Work out the finished part from the listing and answer in its coordinate system (mm). Face numbers are marked on the shaded views. Round coordinates to 2 decimals unless told otherwise and drop trailing zeros. Order: outer loops, then holes, each group sorted by start corner. A loop starts at its lowest first (then second) coordinate and runs counter-clockwise, first axis right, second up. Notation, with made-up numbers: (76, -18) - (96, -18) arc R22 ccw to (96, 15) - close; hole circle Ø8 at (59.5, 9). An arc over 180 degrees is marked (long way). Put each result on its own line as item: value.
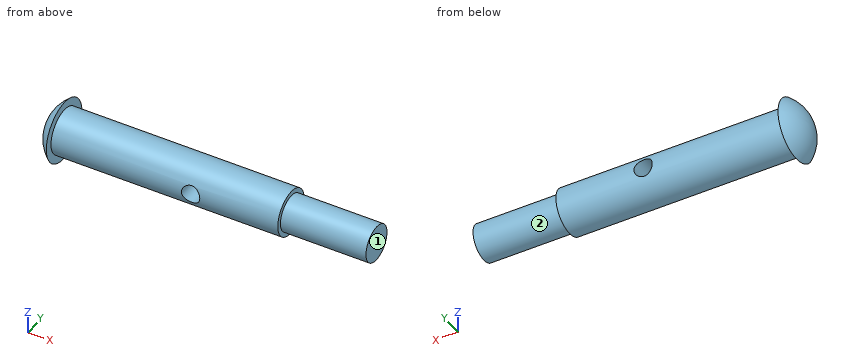
```python
from build123d import *

# Parameters (mm, degrees)
SKETCH4_R               = 0.9906
CUT_EXTRUDE1_DEPTH      = 4.3274
CUT_EXTRUDE1_DEPTH_BACK = 4.3274


with BuildPart() as part:
    # Sketch1 → Revolve1 (revolve)
    with BuildSketch(Plane.XY):
        with BuildLine():
            Line((0, 3.3274), (0, 2.45745))
            Line((0, 2.45745), (24.511, 2.45745))
            Line((24.511, 2.45745), (24.511, 1.96215))
            Line((24.511, 1.96215), (33.7566, 1.96215))
            Line((33.7566, 1.96215), (33.7566, 0))
            Line((33.7566, 0), (-1.651, 0))
            ThreePointArc((-1.651, 0), (-1.21556162, 1.857242025), (0, 3.3274))
        make_face()
    revolve(axis=Axis((0, 0, 0), (1, 0, 0)))

    # Sketch4 → Cut-Extrude1 (cut, two sides)
    with BuildSketch(Plane(origin=(0, 0, 0), x_dir=(1, 0, 0), z_dir=(0, 1, 0))) as cut_extrude1_sk:
        with Locations((15.0876, 0)):
            Circle(SKETCH4_R)
    extrude(amount=CUT_EXTRUDE1_DEPTH, mode=Mode.SUBTRACT)
    extrude(cut_extrude1_sk.sketch, amount=-CUT_EXTRUDE1_DEPTH_BACK, mode=Mode.SUBTRACT)


solid = part.part
```
1) A cutting plane is placed at D-D on x = 25.5. Write down the section's boundary in (y, z), then the cut area to 3 significant figures.
Findings below:
outline: circle Ø3.92 at (0, 0)
area: 12.1 mm2
2) A cutting plane is placed at B-B on y = 0.5. Write down the section's boundary in (x, z).
Findings below:
outline: (0, -3.29) - (0, -2.41) - (24.51, -2.41) - (24.51, -1.9) - (33.76, -1.9) - (33.76, 1.9) - (24.51, 1.9) - (24.51, 2.41) - (0, 2.41) - (0, 3.29) arc R4.15 ccw to start; hole circle Ø1.98 at (15.09, 0)
3) For a pull along X with two mould halves and no side action, classify the marked faces 1 and 2 as pulls with the +X half, pulls with the -X half, needs draft (parallel to the pull), parting line crosses it, or undercut.
Findings below:
face 1: pulls with the +X half
face 2: needs draft
4) A cutting plane is placed at C-C on x = 20. Write down the section's boundary in (y, z).
Findings below:
outline: circle Ø4.91 at (0, 0)
5) Given pin 1 Ø3 at (x, y) = (16, -1) entering from +Z; pin 2 Ø1.5 at (x, y) = (5, 0.5) entering from -Z; pin 3 Ø1.5 at (x, y) = (28.5, 2) entering from +Z, each flat-ended and moving along its own axis, determine where each tip first touches the part or whether it passes through.
Findings below:
pin 1: stops at z = 2.46
pin 2: stops at z = -2.46
pin 3: stops at z = 1.51
6) A cutting plane is placed at A-A on z = 0. Write down the section's boundary in (x, y).
Findings below:
outline: (0, -3.33) - (0, -2.46) - (14.1, -2.46) - (14.1, 2.46) - (0, 2.46) - (0, 3.33) arc R4.18 ccw to start; (16.08, -2.46) - (24.51, -2.46) - (24.51, -1.96) - (33.76, -1.96) - (33.76, 1.96) - (24.51, 1.96) - (24.51, 2.46) - (16.08, 2.46) - close
7) Straight lines are drawn through the part: L1, parallel to Z at x = 15, y = 1.75; L2, parallel to Y at x = 22, z = 0; L3, parallel to X at y = 1.5, z = -0.5. For each, find the intervals that lie inside material, in ascending order. Write a range as from..to.
Findings below:
L1: z = -1.73..-0.99, 0.99..1.73
L2: y = -2.46..2.46
L3: x = -1.34..14.23, 15.94..33.76
